Input: part model. Units: mm. Frame: model coordinates. A direction names the side the tool comes from. Round coordinates to 2 decimals unless told otherwise and drop trailing zeros. Write each loop counter-clockwise with the first axis right and the second up, starting at its lowest first coordinate (ties: lowest second). Pieces come first, ordered by that corner, then holes. Notation, with made-up numbers: (24, 72.25) -> (83, 72.25) arc R7 cw to (83, 77.25) -> close; hole circle Ø2 at (29.25, -25). An arc over 180 degrees is marked (long way). Write item = value, one per line.
```python
from build123d import *

# Parameters (mm, degrees)
SKETCH_1_R                = 115
SKETCH_1_R_2              = 105
EXTRUDE_1_DEPTH           = 5
SKETCH_4_R                = 2.5
CUT_EXTRUDE_1_DEPTH       = 33.934862746
EXTRUDE_2_DEPTH           = 5
HOLE_WIZARD_1_D           = 4.5
HOLE_WIZARD_1_CBORE_D     = 6
HOLE_WIZARD_1_CBORE_DEPTH = 3
SKETCH_9_R                = 2.25
SKETCH_9_R_2              = 1.9
EXTRUDE_3_DEPTH           = 5
EXTRUDE_4_DEPTH           = 5
HOLE_WIZARD_2_D           = 4.5
HOLE_WIZARD_2_CBORE_D     = 6
HOLE_WIZARD_2_CBORE_DEPTH = 3
SKETCH_13_R               = 2.25
SKETCH_13_R_2             = 1.9
EXTRUDE_5_DEPTH           = 5
SKETCH_14_W               = 562.038590931
SKETCH_14_H               = 462.09177453
CUT_EXTRUDE_4_DEPTH       = 163.29776757
SKETCH_15_W               = 637.223239982
SKETCH_15_H               = 375.31186697
CUT_EXTRUDE_5_DEPTH       = 202.710100717


with BuildPart() as part:
    # 草图1 → 凸台-拉伸1 (new body, symmetric)
    with BuildSketch(Plane.XY):
        Circle(SKETCH_1_R)
        Circle(SKETCH_1_R_2, mode=Mode.SUBTRACT)
    extrude(amount=EXTRUDE_1_DEPTH, both=True)

    # 扫描1: sweep along a path in 草图2
    with BuildLine(Plane(origin=(0, 0, 0), x_dir=(1, 0, 0), z_dir=(0, 1, 0))) as sweep_1_path:
        Line((-130, -355), (-156.694693778, -281.656931626))
        ThreePointArc((-156.694693778, -281.656931626), (-157.1458451, -279.97321197), (-157.29776757, -278.236730193))
        Line((-157.29776757, -278.236730193), (-157.29776757, -10))
        ThreePointArc((-157.29776757, -10), (-154.368835382, -2.928932188), (-147.29776757, 0))
        Line((-147.29776757, 0), (-115, 0))
        Line((-115, 0), (-106.681302201, 0))
    # 草图3 → 扫描1 (sweep)
    with BuildSketch(Plane(origin=(-130, 0, 355), x_dir=(0.939692621, 0, -0.342020143), z_dir=(0.342020143, 0, 0.939692621))):
        Polygon((-5, -15), (5, -15), (5, -11.5), (2, -11.5), (2, 11.5), (5, 11.5), (5, 15), (-5, 15), align=None)
    sweep_1 = sweep(path=sweep_1_path.line)

    # 草图4 → 切除-拉伸1 (cut, through all)
    with BuildSketch(Plane(origin=(-227.008304281, 0, 82.624265689), x_dir=(-0.342020143, 0, -0.939692621), z_dir=(0.939692621, 0, -0.342020143))):
        with Locations((-274.128261747, 6.75)):
            Circle(SKETCH_4_R)
        with Locations((-274.128261747, -6.75)):
            Circle(SKETCH_4_R)
    cut_extrude_1 = extrude(amount=-CUT_EXTRUDE_1_DEPTH, mode=Mode.SUBTRACT)

    # 镜向1: 扫描1, 切除-拉伸1 across plane
    add(sweep_1.mirror(Plane(origin=(0, 0, 0), x_dir=(0, 0, 1), z_dir=(1, 0, 0))))
    add(cut_extrude_1.mirror(Plane(origin=(0, 0, 0), x_dir=(0, 0, 1), z_dir=(1, 0, 0))), mode=Mode.SUBTRACT)

    # 草图6 → 凸台-拉伸2 (add, symmetric)
    with BuildSketch(Plane(origin=(0, 0, 0), x_dir=(0, 0, -1), z_dir=(1, 0, 0))):
        with BuildLine():
            Line((-5, 115), (-5, 125))
            ThreePointArc((-5, 125), (0, 130), (5, 125))
            Line((5, 125), (5, 115))
            Line((5, 115), (5, 112.136445143))
            Line((5, 112.136445143), (-5, 112.136445143))
            Line((-5, 112.136445143), (-5, 115))
        make_face()
    extrude_2 = extrude(amount=EXTRUDE_2_DEPTH, both=True)

    # 镜向2: 凸台-拉伸2 across plane
    add(extrude_2.mirror(Plane.ZX))

    # 孔1 (through all)
    with Locations(Plane(origin=(5, 0, 0), x_dir=(0, 0, -1), z_dir=(1, 0, 0))):
        with Locations((0, 124.156343107), (0, -125)):
            CounterBoreHole(HOLE_WIZARD_1_D / 2, HOLE_WIZARD_1_CBORE_D / 2, HOLE_WIZARD_1_CBORE_DEPTH)

    # 草图9 → 凸台-拉伸3 (add)
    with BuildSketch(Plane.ZY.offset(5)):
        with Locations((0, 124.156343107)):
            Circle(SKETCH_9_R)
        with Locations((0, 124.156343107)):
            Circle(SKETCH_9_R_2, mode=Mode.SUBTRACT)
        with Locations((0, -125)):
            Circle(SKETCH_9_R)
        with Locations((0, -125)):
            Circle(SKETCH_9_R_2, mode=Mode.SUBTRACT)
    extrude(amount=-EXTRUDE_3_DEPTH)

    # 草图10 → 凸台-拉伸4 (add, symmetric)
    with BuildSketch(Plane.XY.offset(155)):
        with BuildLine():
            Line((-162.29776757, 15), (-152.29776757, 15))
            Line((-152.29776757, 15), (-152.29776757, 20))
            ThreePointArc((-152.29776757, 20), (-157.29776757, 25), (-162.29776757, 20))
            Line((-162.29776757, 20), (-162.29776757, 15))
        make_face()
        with BuildLine():
            Line((-152.29776757, -15), (-152.29776757, -20))
            ThreePointArc((-152.29776757, -20), (-157.29776757, -25), (-162.29776757, -20))
            Line((-162.29776757, -20), (-162.29776757, -15))
            Line((-162.29776757, -15), (-152.29776757, -15))
        make_face()
        with BuildLine():
            Line((162.29776757, -15), (152.29776757, -15))
            Line((152.29776757, -15), (152.29776757, -20))
            ThreePointArc((152.29776757, -20), (157.29776757, -25), (162.29776757, -20))
            Line((162.29776757, -20), (162.29776757, -15))
        make_face()
        with BuildLine():
            Line((152.29776757, 15), (152.29776757, 20))
            ThreePointArc((152.29776757, 20), (157.29776757, 25), (162.29776757, 20))
            Line((162.29776757, 20), (162.29776757, 15))
            Line((162.29776757, 15), (152.29776757, 15))
        make_face()
    extrude(amount=EXTRUDE_4_DEPTH, both=True)

    # 孔2 (through all)
    with Locations(Plane.XY.offset(160)):
        with Locations((-157.29776757, 20), (-157.29776757, -20), (157.29776757, 20), (157.29776757, -20)):
            CounterBoreHole(HOLE_WIZARD_2_D / 2, HOLE_WIZARD_2_CBORE_D / 2, HOLE_WIZARD_2_CBORE_DEPTH)

    # 草图13 → 凸台-拉伸5 (add)
    with BuildSketch(Plane(origin=(0, 0, 150), x_dir=(-1, 0, 0), z_dir=(0, 0, -1))):
        with Locations((-157.29776757, 20)):
            Circle(SKETCH_13_R)
        with Locations((-157.29776757, 20)):
            Circle(SKETCH_13_R_2, mode=Mode.SUBTRACT)
        with Locations((-157.29776757, -20)):
            Circle(SKETCH_13_R)
        with Locations((-157.29776757, -20)):
            Circle(SKETCH_13_R_2, mode=Mode.SUBTRACT)
        with Locations((157.29776757, -20)):
            Circle(SKETCH_13_R)
        with Locations((157.29776757, -20)):
            Circle(SKETCH_13_R_2, mode=Mode.SUBTRACT)
        with Locations((157.29776757, 20)):
            Circle(SKETCH_13_R)
        with Locations((157.29776757, 20)):
            Circle(SKETCH_13_R_2, mode=Mode.SUBTRACT)
    extrude(amount=-EXTRUDE_5_DEPTH)

    # 草图14 → 切除-拉伸4 (cut, through all)
    with BuildSketch(Plane(origin=(0, 0, 0), x_dir=(0, 0, -1), z_dir=(1, 0, 0))):
        with Locations((-153.139864812, -31.152254463)):
            Rectangle(SKETCH_14_W, SKETCH_14_H)
    extrude(amount=CUT_EXTRUDE_4_DEPTH, mode=Mode.SUBTRACT)

    # 草图15 → 切除-拉伸5 (cut, through all)
    with BuildSketch(Plane.XY.offset(155)):
        Rectangle(SKETCH_15_W, SKETCH_15_H)
    extrude(amount=CUT_EXTRUDE_5_DEPTH, mode=Mode.SUBTRACT)


solid = part.part
```
1) First-contact query: P1, Ø4.5, axis at y = -125, z = 0, coming from the +X side; P2, Ø7, axis at y = 17, z = 63.5, coming from the +X side; P3, Ø4.5, axis at x = -157.3, y = 20, coming from the -Z side; P4, Ø5, axis at y = 123.5, z = 0, coming from the -X side. Flat tips, straight axial feed; report the tip coordinate or a pass-through.
Solutions:
P1 = 0
P2 = -152.3
P3 = 150
P4 = -5
2) Draft query along X for faces 5 (the face through (-152.298, -13, 81)), 6 (the face through (-155, -11.5, 63)), 7 (the face through (-157.4, 17.8, 150)). Return one class per face: +X half, -X half, draft (parallel to the pull), parting line (faces both ways), or undercut.
Solutions:
face_5 = +X half
face_6 = undercut
face_7 = draft
3) Access query for faces 1 (the face through (-153.02, 0.16, 4.41)), 2 (the face through (-154, -15, 62)), 3 (the face through (-157.2, -17.7, 150)), 4 (the face through (-5, -122.6, -0.1)). Directions: +Z, -Z, +X, -X, +Y, -Y. A direction counts if a zero-diameter tool reaches every point of the face in a straight line with its end or side. Return the directions, or none.
Solutions:
face_1 = +Z
face_2 = -Z, -X, -Y
face_3 = -Z, +X, -X, -Y
face_4 = +Z, -Z, -X, -Y
4) Cut plane C-C (x = -119). Return the cut outline in (y, z).
Solutions:
outline = (-15, -5) -> (15, -5) -> (15, 5) -> (11.5, 5) -> (11.5, 2) -> (-11.5, 2) -> (-11.5, 5) -> (-15, 5) -> close
5) Cut plane D-D (y = 0). Return the cut outline in (x, z).
Solutions:
outline = (-162.3, 10) arc R15 ccw to (-147.3, -5) -> (-105, -5) -> (-105, 5) -> (-115, 5) -> (-115, 2) -> (-147.3, 2) arc R8 cw to (-155.3, 10) -> (-155.3, 155) -> (-162.3, 155) -> close
6) Cut plane B-B (z = 138). Return the cut outline in (x, y).
Solutions:
outline = (-162.3, -15) -> (-152.3, -15) -> (-152.3, -11.5) -> (-155.3, -11.5) -> (-155.3, 11.5) -> (-152.3, 11.5) -> (-152.3, 15) -> (-162.3, 15) -> close
7) Cut plane A-A (x = -97.5). Return the cut outline in (y, z), and give its area (3 significant figures).
Solutions:
outline = (-60.98, -5) -> (-38.97, -5) -> (-38.97, 5) -> (-60.98, 5) -> close; (38.97, -5) -> (60.98, -5) -> (60.98, 5) -> (38.97, 5) -> close
area = 440 mm^2
8) Line query: L1, parallel to Y at x = -2, z = 0; L2, parallel to Y at x = -155, z = 37.5; L3, parallel to Z at x = -2.65, y = -125. Output: solid intervals per line, ascending. Write a range as from..to.
Solutions:
L1 = -130..-126.9, -123.1..-104.98, 104.98..122.26, 126.06..130
L2 = -15..-11.5, 11.5..15
L3 = -5..-1.9, 1.9..5
